Geometry check sheet. Reference: drawing and pictorial views, mm from the part's lowest x, y, z. A direction names the side the tool comes from. Round coordinates to 2 decimals unless told otherwise and drop trailing zeros. Order: outer loops, then holes, each group sorted by start corner. A loop starts at its lowest first (then second) coordinate and runs counter-clockwise, first axis right, second up.
(1) Release check for a two-part mould opening along X. For the marked faces 1, 2, 3 and 4 record: +X half, -X half, draft (parallel to the pull), parting line (faces both ways), or undercut.
(2) Material ranges on line 1 along X through (y, z) = (40, 18.85); line 2 along X through (y, z) = (40, 15.95); line 3 along Y through (x, z) = (15, 19.55), recorded low to high.
(3) Sectioned sample at A-A (y = 40). Record the boundary of the cut face in (x, z), plus the area to 3 significant figures.
(4) Go/stop test with flat-tipped pins: pin 1 (4 mm diameter, centred on x = 29, y = 33, fed in from -Z); pin 2 (3 mm diameter, centred on x = 13, y = 38, fed in from +Z); pin 3 (3.5 mm diameter, centred on x = 45, y = 40, fed in from +Z); pin 4 (1.6 mm diameter, centred on x = 10, z = 1, fed in from +Y). Record where each tip stops, or that it passes through.
(5) Sectioned sample at C-C (x = 53). Record the boundary of the cut face in (y, z), plus the area to 3 significant figures.
(6) Sectioned sample at B-B (z = 7). Record the boundary of the cut face in (x, y).
(7) Sectioned sample at D-D (x = 13). Record the boundary of the cut face in (y, z).
(8) Set-up check for the marked faces 5, 6, 7, 8 and 9: record each of +Z, -Z, +X, -X, +Y, -Y from which the full face is reachable in a straight line by a thin tool's end or side.
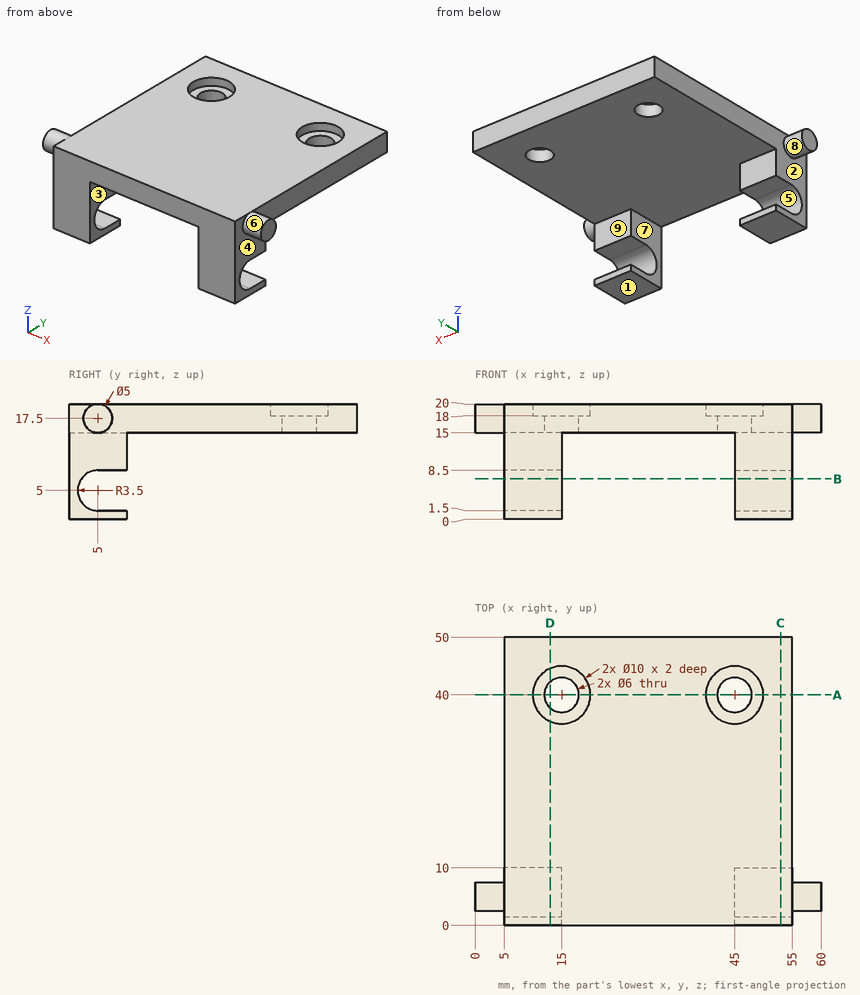
Answer below:
1. face 1: draft
1. face 2: -X half
1. face 3: undercut
1. face 4: +X half
2. line 1: x = 5 to 10, 20 to 40, 50 to 55
2. line 2: x = 5 to 12, 18 to 42, 48 to 55
2. line 3: y = 0 to 35, 45 to 50
3. outline: (5, 15) - (12, 15) - (12, 18) - (10, 18) - (10, 20) - (5, 20) - close; (18, 15) - (42, 15) - (42, 18) - (40, 18) - (40, 20) - (20, 20) - (20, 18) - (18, 18) - close; (48, 15) - (55, 15) - (55, 20) - (50, 20) - (50, 18) - (48, 18) - close
3. area: 174 mm2
4. pin 1: stops at z = 15
4. pin 2: stops at z = 18
4. pin 3: passes through
4. pin 4: stops at y = 10
5. outline: (0, 0) - (10, 0) - (10, 1.5) - (5, 1.5) arc R3.5 cw to (5, 8.5) - (10, 8.5) - (10, 15) - (50, 15) - (50, 20) - (0, 20) - close
5. area: 346 mm2
6. outline: (5, 0) - (15, 0) - (15, 2.13) - (5, 2.13) - close; (45, 0) - (55, 0) - (55, 2.13) - (45, 2.13) - close
7. outline: (0, 0) - (10, 0) - (10, 1.5) - (5, 1.5) arc R3.5 cw to (5, 8.5) - (10, 8.5) - (10, 15) - (37.76, 15) - (37.76, 18) - (35.42, 18) - (35.42, 20) - (0, 20) - close; (42.24, 15) - (50, 15) - (50, 20) - (44.58, 20) - (44.58, 18) - (42.24, 18) - close
8. face 5: +X, -X, +Y
8. face 6: +X
8. face 7: -Z, +Y, -Y
8. face 8: -X
8. face 9: -Z, +X, -X, +Y
